Could you check a few things on this model? Use its own coordinates, in mm. Face numbers are marked on the shaded views. A direction names the side the tool comes from. Round coordinates to 2 decimals unless told otherwise and drop trailing zeros. Loops run counter-clockwise (first coordinate to the right, second up) from the corner with the lowest first, then second, coordinate; pieces in that order, holes last. Notation, with made-up numbers: (-39, -14.75) - (-19, -14.75) arc R16 ccw to (-19, 12.25) - close; hole circle Ø8 at (-0.75, 53). An arc over 180 degrees is marked (long way). Put each result on its own line as item: value. Start each with the question number.
from build123d import *

# Parameters (mm, degrees)
F0_W         = 145.6760466099
F0_H         = 100.0369116664
F0_W_2       = 138.8105116785
F0_H_2       = 92.9268449545
F1_DEPTH     = 25.4
F2_T         = -2.54
F3_T1_DEPTH  = 171.0760466099
F3_T3_DEPTH  = 125.4369116664
F4_DEPTH     = 25.4
F5_T1_DEPTH  = 58.42
F5_S5_W      = 5.08
F5_S5_H      = 5.08
F5_T6_DEPTH  = 5.08
F5_S11_W     = 5.08
F5_S11_H     = 5.08
F5_T12_DEPTH = 5.08


# Not quite as in the source:
# - a fillet or chamfer that OpenCascade refuses, or shapes differently, is made with other operations: its cross-section is extruded or revolved along the edge and cut away or added


with BuildPart() as f1:
    # F0 (on Front) → F1 (new body)
    with BuildSketch(Plane.XZ):
        with Locations((-20.1583206654, 2.9303953052)):
            Rectangle(F0_W, F0_H)
        with Locations((-20.7056272775, 3.0381605029)):
            Rectangle(F0_W_2, F0_H_2, mode=Mode.SUBTRACT)
        with Locations((-20.7056272775, 3.0381605029)):
            Rectangle(F0_W_2, F0_H_2)
    extrude(amount=F1_DEPTH)

    # F2
    f2_openings = [f1.faces().sort_by_distance(p)[0] for p in [
        (-20.158321, -25.4, 2.930395),
        (-92.996344, -12.7, 2.930395),
    ]]
    offset(amount=F2_T, openings=f2_openings)

    # F3: fillet of radius 5.08 on 4 edges, made by hand

    # F3_s2 → F3_t1 (cut)
    with BuildSketch(Plane.YZ.offset(-105.6963439703)):
        with BuildLine():
            ThreePointArc((-5.08, 52.9488511384), (-1.4878975516, 51.4609535868), (0, 47.8688511384))
            Line((0, 47.8688511384), (0, 52.9488511384))
            Line((0, 52.9488511384), (-5.08, 52.9488511384))
        make_face()
        with BuildLine():
            ThreePointArc((-5.08, -47.088060528), (-1.4878975516, -45.6001629765), (0, -42.008060528))
            Line((0, -42.008060528), (0, -47.088060528))
            Line((0, -47.088060528), (-5.08, -47.088060528))
        make_face()
    extrude(amount=F3_T1_DEPTH, mode=Mode.SUBTRACT)

    # F3_s4 → F3_t3 (cut)
    with BuildSketch(Plane.XY.offset(-59.788060528)):
        with BuildLine():
            ThreePointArc((-87.9163439703, 0), (-91.5084464187, -1.4878975516), (-92.9963439703, -5.08))
            Line((-92.9963439703, -5.08), (-92.9963439703, 0))
            Line((-92.9963439703, 0), (-87.9163439703, 0))
        make_face()
        with BuildLine():
            ThreePointArc((52.6797026396, -5.08), (51.191805088, -1.4878975516), (47.5997026396, 0))
            Line((47.5997026396, 0), (52.6797026396, 0))
            Line((52.6797026396, 0), (52.6797026396, -5.08))
        make_face()
    extrude(amount=F3_T3_DEPTH, mode=Mode.SUBTRACT)

    # F4 (add): a face of the model
    f4_faces = [f1.faces().sort_by_distance(p)[0] for p in [
        (-20.1583206654, -25.4, 51.1816812469),
    ]]
    extrude(f4_faces, amount=F4_DEPTH)

    # F5: fillet of radius 5.08 on 2 edges, made by hand

    # F5_s2 → F5_t1 (cut)
    with BuildSketch(Plane.XZ.offset(5.08)):
        with BuildLine():
            ThreePointArc((52.6797026396, 47.8688511384), (51.191805088, 51.4609535868), (47.5997026396, 52.9488511384))
            Line((47.5997026396, 52.9488511384), (52.6797026396, 52.9488511384))
            Line((52.6797026396, 52.9488511384), (52.6797026396, 47.8688511384))
        make_face()
        with BuildLine():
            ThreePointArc((47.5997026396, -47.088060528), (51.191805088, -45.6001629765), (52.6797026396, -42.008060528))
            Line((52.6797026396, -42.008060528), (52.6797026396, -47.088060528))
            Line((52.6797026396, -47.088060528), (47.5997026396, -47.088060528))
        make_face()
    extrude(amount=F5_T1_DEPTH, mode=Mode.SUBTRACT)


with BuildPart() as f5_tool4:
    # F5_s5 → F5_t6 (new body)
    with BuildSketch(Plane.XY.offset(-42.008060528)):
        with Locations((50.1397026396, -2.54)):
            Rectangle(F5_S5_W, F5_S5_H)
    extrude(amount=-F5_T6_DEPTH)

    # F5_s7 → F5_t8 (revolve, cut)
    with BuildSketch(Plane(origin=(47.5997026396, -5.08, -42.008060528), x_dir=(-0.7071067812, -0.7071067812, 0), z_dir=(0.7071067812, -0.7071067812, 0))):
        with BuildLine():
            ThreePointArc((0, -5.08), (5.08, 0), (0, 5.08))
            Line((0, 5.08), (0, -5.08))
        make_face()
    revolve(axis=Axis((47.5997026396, -5.08, -42.008060528), (0, 0, -1)), mode=Mode.SUBTRACT)


with BuildPart() as f1_1:
    add(f1.part)

    # F5_t3: cut F5_tool4
    add(f5_tool4.part, mode=Mode.SUBTRACT)


with BuildPart() as f5_tool10:
    # F5_s11 → F5_t12 (new body)
    with BuildSketch(Plane.YZ.offset(47.5997026396)):
        with Locations((-2.54, 50.4088511384)):
            Rectangle(F5_S11_W, F5_S11_H)
    extrude(amount=F5_T12_DEPTH)

    # F5_s13 → F5_t14 (revolve, cut)
    with BuildSketch(Plane(origin=(47.5997026396, -5.08, 47.8688511384), x_dir=(0, -0.7071067812, -0.7071067812), z_dir=(0, -0.7071067812, 0.7071067812))):
        with BuildLine():
            ThreePointArc((0, -5.08), (5.08, 0), (0, 5.08))
            Line((0, 5.08), (0, -5.08))
        make_face()
    revolve(axis=Axis((47.5997026396, -5.08, 47.8688511384), (1, 0, 0)), mode=Mode.SUBTRACT)


with BuildPart() as f1_2:
    add(f1_1.part)

    # F5_t9: cut F5_tool10
    add(f5_tool10.part, mode=Mode.SUBTRACT)


solid = f1_2.part
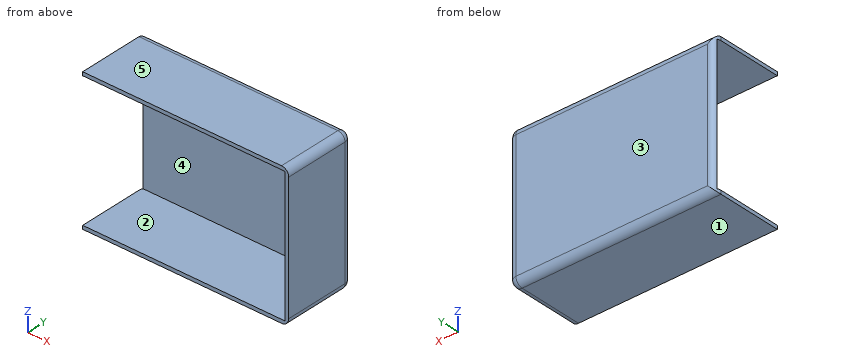
Item 1: I need wall thicknesses on line 1 (Z direction, x = -7.5, y = -42.5); line 2 (Y direction, x = 25, z = -9.5); line 3 (X direction, y = -38, z = -33). Which ranges of each line are inside material? Lowest first, please. Write a range as from..to.
Item 2: Will this pin go through, and if not, where does the flat tip stop? P1, Ø10, axis at y = -24, z = 35, coming from the -X side.
Item 3: On a 3-axis mill with a long thin cutter (end or side, diameter ignored), from which of +Z, -Z, +X, -X, +Y, -Y can I reach the whole of each face in a straight line? I mean the marked faces 1 and 2. Say none if no direction works.
Item 4: Suppose I cut it at C-C, the plane x = -64.5. List the corners of the cut face in (y, z) for me.
Item 5: Suppose I cut it at A-A, the plane y = -24. List the corners of the cut face in (x, z) for me.
Item 6: Suppose I cut it at B-B, the plane z = -11. List the corners of the cut face in (x, y) for me, then the cut area to 3 significant figures.
Item 7: Thinking about a two-plate mould opening in Z: for the marked faces 3, 4 and 5, which applies, released by +Z, released by -Z, zero draft, split by the parting line, or undercut?
Numbers:
1. line 1: -47.09..-44.55, 50.41..52.95
1. line 2: -2.54..0
1. line 3: 50.14..52.68
2. P1: x = 50.14
3. face 1: -Z, +X, -X, +Y, -Y
3. face 2: -X, -Y
4. outline: (-50.8, -47.09) - (-5.08, -47.09) arc R5.08 ccw to (0, -42.01) - (0, 47.87) arc R5.08 ccw to (-5.08, 52.95) - (-50.8, 52.95) - (-50.8, 50.41) - (-2.54, 50.41) - (-2.54, -44.55) - (-50.8, -44.55) - close
5. outline: (-93, -47.09) - (47.6, -47.09) arc R5.08 ccw to (52.68, -42.01) - (52.68, 47.87) arc R5.08 ccw to (47.6, 52.95) - (-93, 52.95) - (-93, 50.41) - (50.14, 50.41) - (50.14, -44.55) - (-93, -44.55) - close
6. outline: (-92.32, -2.54) - (50.14, -2.54) - (50.14, -50.8) - (52.68, -50.8) - (52.68, -5.08) arc R5.08 ccw to (47.6, 0) - (-87.92, 0) arc R5.08 ccw to start
6. area: 482 mm^2
7. face 3: zero draft
7. face 4: undercut
7. face 5: released by +Z
